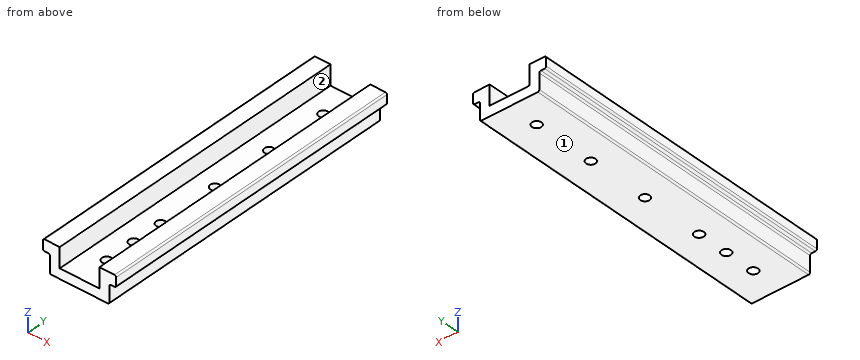
```python
from build123d import *

# Parameters (mm, degrees)
BOSS_EXTRUDE1_DEPTH = 100
CUT_EXTRUDE1_REACH  = 103.133
SKETCH2_R           = 1.5


with BuildPart() as part:
    # Sketch1 → Boss-Extrude1 (new body)
    with BuildSketch(Plane(origin=(0, 0, 0), x_dir=(1, 0, 0), z_dir=(0, 1, 0))):
        with BuildLine():
            Line((11.2078125, 0), (6.35, 0))
            Line((6.35, 0), (6.35, 6.35))
            Line((6.35, 6.35), (-6.35, 6.35))
            Line((-6.35, 6.35), (-6.35, 0))
            Line((-6.35, 0), (-11.2078125, 0))
            ThreePointArc((-11.2078125, 0), (-11.561365891, 0.146446609), (-11.7078125, 0.5))
            Line((-11.7078125, 0.5), (-11.7078125, 3.071875))
            ThreePointArc((-11.7078125, 3.071875), (-11.561365891, 3.425428391), (-11.2078125, 3.571875))
            Line((-11.2078125, 3.571875), (-10.025, 3.571875))
            ThreePointArc((-10.025, 3.571875), (-9.671446609, 3.718321609), (-9.525, 4.071875))
            Line((-9.525, 4.071875), (-9.525, 9.025))
            ThreePointArc((-9.525, 9.025), (-9.378553391, 9.378553391), (-9.025, 9.525))
            Line((-9.025, 9.525), (9.025, 9.525))
            ThreePointArc((9.025, 9.525), (9.378553391, 9.378553391), (9.525, 9.025))
            Line((9.525, 9.025), (9.525, 4.071875))
            ThreePointArc((9.525, 4.071875), (9.671446609, 3.718321609), (10.025, 3.571875))
            Line((10.025, 3.571875), (11.2078125, 3.571875))
            ThreePointArc((11.2078125, 3.571875), (11.561365891, 3.425428391), (11.7078125, 3.071875))
            Line((11.7078125, 3.071875), (11.7078125, 0.5))
            ThreePointArc((11.7078125, 0.5), (11.561365891, 0.146446609), (11.2078125, 0))
        make_face()
    extrude(amount=BOSS_EXTRUDE1_DEPTH)

    # Sketch2 → Cut-Extrude1 (cut, up to next)
    with BuildSketch(Plane(origin=(0, 0, -9.525), x_dir=(-1, 0, 0), z_dir=(0, 0, -1)), mode=Mode.PRIVATE) as cut_extrude1_sk1:
        with Locations((0, 10)):
            Circle(SKETCH2_R)
    cut_extrude1_tool1 = extrude(cut_extrude1_sk1.sketch, amount=-CUT_EXTRUDE1_REACH, mode=Mode.PRIVATE) & part.part
    # Sketch2 → Cut-Extrude1 (cut, up to next)
    with BuildSketch(Plane(origin=(0, 0, -9.525), x_dir=(-1, 0, 0), z_dir=(0, 0, -1)), mode=Mode.PRIVATE) as cut_extrude1_sk2:
        with Locations((0, 20)):
            Circle(SKETCH2_R)
    cut_extrude1_tool2 = extrude(cut_extrude1_sk2.sketch, amount=-CUT_EXTRUDE1_REACH, mode=Mode.PRIVATE) & part.part
    # Sketch2 → Cut-Extrude1 (cut, up to next)
    with BuildSketch(Plane(origin=(0, 0, -9.525), x_dir=(-1, 0, 0), z_dir=(0, 0, -1)), mode=Mode.PRIVATE) as cut_extrude1_sk3:
        with Locations((0, 30)):
            Circle(SKETCH2_R)
    cut_extrude1_tool3 = extrude(cut_extrude1_sk3.sketch, amount=-CUT_EXTRUDE1_REACH, mode=Mode.PRIVATE) & part.part
    # Sketch2 → Cut-Extrude1 (cut, up to next)
    with BuildSketch(Plane(origin=(0, 0, -9.525), x_dir=(-1, 0, 0), z_dir=(0, 0, -1)), mode=Mode.PRIVATE) as cut_extrude1_sk4:
        with Locations((0, 50)):
            Circle(SKETCH2_R)
    cut_extrude1_tool4 = extrude(cut_extrude1_sk4.sketch, amount=-CUT_EXTRUDE1_REACH, mode=Mode.PRIVATE) & part.part
    # Sketch2 → Cut-Extrude1 (cut, up to next)
    with BuildSketch(Plane(origin=(0, 0, -9.525), x_dir=(-1, 0, 0), z_dir=(0, 0, -1)), mode=Mode.PRIVATE) as cut_extrude1_sk5:
        with Locations((0, 70)):
            Circle(SKETCH2_R)
    cut_extrude1_tool5 = extrude(cut_extrude1_sk5.sketch, amount=-CUT_EXTRUDE1_REACH, mode=Mode.PRIVATE) & part.part
    # Sketch2 → Cut-Extrude1 (cut, up to next)
    with BuildSketch(Plane(origin=(0, 0, -9.525), x_dir=(-1, 0, 0), z_dir=(0, 0, -1)), mode=Mode.PRIVATE) as cut_extrude1_sk6:
        with Locations((0, 90)):
            Circle(SKETCH2_R)
    cut_extrude1_tool6 = extrude(cut_extrude1_sk6.sketch, amount=-CUT_EXTRUDE1_REACH, mode=Mode.PRIVATE) & part.part
    add(cut_extrude1_tool1.solids().sort_by_distance((0, 10, -9.525))[0], mode=Mode.SUBTRACT)
    add(cut_extrude1_tool2.solids().sort_by_distance((0, 20, -9.525))[0], mode=Mode.SUBTRACT)
    add(cut_extrude1_tool3.solids().sort_by_distance((0, 30, -9.525))[0], mode=Mode.SUBTRACT)
    add(cut_extrude1_tool4.solids().sort_by_distance((0, 50, -9.525))[0], mode=Mode.SUBTRACT)
    add(cut_extrude1_tool5.solids().sort_by_distance((0, 70, -9.525))[0], mode=Mode.SUBTRACT)
    add(cut_extrude1_tool6.solids().sort_by_distance((0, 90, -9.525))[0], mode=Mode.SUBTRACT)


solid = part.part
```
Design review of the part built by this model. Coordinates are the model's own, in mm. Face numbers are marked on the shaded views. A direction names the side the tool comes from. Coordinates: 2 decimals unless noted, no trailing zeros. Order: outer loops, then holes, each group sorted by start corner. A loop starts at its lowest first (then second) coordinate and runs counter-clockwise, first axis right, second up. Notation, with made-up numbers: (11.5, 89) -> (19.5, 89) arc R33 cw to (19.5, 121) -> close; hole circle Ø6 at (6.25, 42.5). An arc over 180 degrees is marked (long way). One line per item, written item: value. Start each with the question number.
Q1. Insertion check: pin 1 Ø0.9 at (x, y) = (10.5, 32.5) entering from -Z; pin 2 Ø2 at (x, y) = (-2.5, 80.5) entering from +Z; pin 3 Ø1.5 at (y, z) = (75.5, -6.5) entering from -X (3 decimals). Each pin has a flat end and moves straight along its axis. Give the tip position at first contact, or say it passes through.
Q2. Take a section at C-C, the plane y = 80. State the section outline as (x, z) points (3 decimals), then the cut area to 3 significant figures.
Q3. For probe 1 along X at (y, z) = (56.5, -4.75) (3 decimals); probe 2 along X at (y, z) = (90, -8.25) (3 decimals); probe 3 along X at (y, z) = (23, -9) (3 decimals), list the stretches that pass through material, from the lowest coordinate up.
Q4. Take a section at A-A, the plane x = 0. State the section outline as (y, z) points (3 decimals), then the cut area to 3 significant figures.
Q5. Take a section at B-B, the plane y = 30. State the section outline as (x, z) points (3 decimals), then the cut area to 3 significant figures.
Q6. Tool access review of the marked faces 1 and 2: name each direction out of +Z, -Z, +X, -X, +Y, -Y from which nothing blocks a thin tool from reaching the whole face with its end or side.
Values follow:
1. pin 1: stops at z = -3.57
1. pin 2: stops at z = -6.35
1. pin 3: stops at x = -9.525
2. outline: (-11.708, -3.072) arc R0.5 ccw to (-11.208, -3.572) -> (-10.025, -3.572) arc R0.5 cw to (-9.525, -4.072) -> (-9.525, -9.025) arc R0.5 ccw to (-9.025, -9.525) -> (9.025, -9.525) arc R0.5 ccw to (9.525, -9.025) -> (9.525, -4.072) arc R0.5 cw to (10.025, -3.572) -> (11.208, -3.572) arc R0.5 ccw to (11.708, -3.072) -> (11.708, -0.5) arc R0.5 ccw to (11.208, 0) -> (6.35, 0) -> (6.35, -6.35) -> (-6.35, -6.35) -> (-6.35, 0) -> (-11.208, 0) arc R0.5 ccw to (-11.708, -0.5) -> close
2. area: 116 mm2
3. probe 1: x = -9.525 to -6.35, 6.35 to 9.525
3. probe 2: x = -9.525 to -1.5, 1.5 to 9.525
3. probe 3: x = -9.525 to 9.525
4. outline: (0, -9.525) -> (8.5, -9.525) -> (8.5, -6.35) -> (0, -6.35) -> close; (11.5, -9.525) -> (18.5, -9.525) -> (18.5, -6.35) -> (11.5, -6.35) -> close; (21.5, -9.525) -> (28.5, -9.525) -> (28.5, -6.35) -> (21.5, -6.35) -> close; (31.5, -9.525) -> (48.5, -9.525) -> (48.5, -6.35) -> (31.5, -6.35) -> close; (51.5, -9.525) -> (68.5, -9.525) -> (68.5, -6.35) -> (51.5, -6.35) -> close; (71.5, -9.525) -> (88.5, -9.525) -> (88.5, -6.35) -> (71.5, -6.35) -> close; (91.5, -9.525) -> (100, -9.525) -> (100, -6.35) -> (91.5, -6.35) -> close
4. area: 260 mm2
5. outline: (-11.708, -3.072) arc R0.5 ccw to (-11.208, -3.572) -> (-10.025, -3.572) arc R0.5 cw to (-9.525, -4.072) -> (-9.525, -9.025) arc R0.5 ccw to (-9.025, -9.525) -> (-1.5, -9.525) -> (-1.5, -6.35) -> (-6.35, -6.35) -> (-6.35, 0) -> (-11.208, 0) arc R0.5 ccw to (-11.708, -0.5) -> close; (1.5, -9.525) -> (9.025, -9.525) arc R0.5 ccw to (9.525, -9.025) -> (9.525, -4.072) arc R0.5 cw to (10.025, -3.572) -> (11.208, -3.572) arc R0.5 ccw to (11.708, -3.072) -> (11.708, -0.5) arc R0.5 ccw to (11.208, 0) -> (6.35, 0) -> (6.35, -6.35) -> (1.5, -6.35) -> close
5. area: 107 mm2
6. face 1: -Z, +X, -X, +Y, -Y
6. face 2: +Z, +Y, -Y
